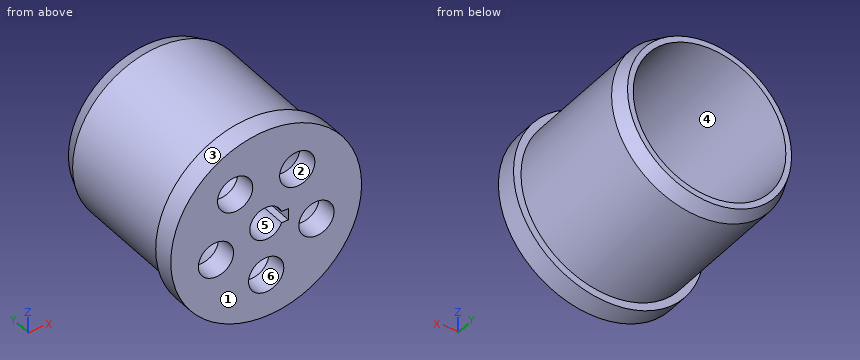
```python
from build123d import *

# Parameters (mm, degrees)
SKETCH1_R           = 41.275
SKETCH1_R_2         = 7.62
BOSS_EXTRUDE1_DEPTH = 9.525
SKETCH2_R           = 38.0365
SKETCH2_R_2         = 33.02
BOSS_EXTRUDE2_DEPTH = 63.5
SKETCH3_R           = 12.7
BOSS_EXTRUDE3_DEPTH = 15.875
CHAMFER1_SIZE       = 6.35
CHAMFER1_SIZE2      = 2.54
SKETCH4_R           = 12.7
BOSS_EXTRUDE4_DEPTH = 6.35
FILLET1_R           = 2.54


with BuildPart() as part:
    # Sketch1 → Boss-Extrude1 (new body)
    with BuildSketch(Plane(origin=(0, 0, 0), x_dir=(1, 0, 0), z_dir=(0, 1, 0))):
        Circle(SKETCH1_R)
        with Locations((-13.436770867, -18.494128491)):
            Circle(SKETCH1_R_2, mode=Mode.SUBTRACT)
        with Locations((13.436770867, -18.494128491)):
            Circle(SKETCH1_R_2, mode=Mode.SUBTRACT)
        with BuildLine():
            Line((9.6, -2.5), (6.64529909, -2.5))
            ThreePointArc((6.64529909, -2.5), (-7.1, 0), (6.64529909, 2.5))
            Line((6.64529909, 2.5), (9.6, 2.5))
            Line((9.6, 2.5), (9.6, -2.5))
        make_face(mode=Mode.SUBTRACT)
        with Locations((-21.741151963, 7.064128491)):
            Circle(SKETCH1_R_2, mode=Mode.SUBTRACT)
        with BuildLine():
            ThreePointArc((0, 15.24), (-7.62, 22.86), (0, 30.48))
            ThreePointArc((0, 30.48), (7.62, 22.86), (0, 15.24))
        make_face(mode=Mode.SUBTRACT)
        with Locations((21.741151963, 7.064128491)):
            Circle(SKETCH1_R_2, mode=Mode.SUBTRACT)
    extrude(amount=BOSS_EXTRUDE1_DEPTH)

    # Sketch2 → Boss-Extrude2 (add)
    with BuildSketch(Plane(origin=(0, 9.525, 0), x_dir=(1, 0, 0), z_dir=(0, 1, 0))):
        Circle(SKETCH2_R)
        Circle(SKETCH2_R_2, mode=Mode.SUBTRACT)
    extrude(amount=BOSS_EXTRUDE2_DEPTH)

    # Sketch3 → Boss-Extrude3 (add)
    with BuildSketch(Plane(origin=(0, 9.525, 0), x_dir=(1, 0, 0), z_dir=(0, 1, 0))):
        Circle(SKETCH3_R)
        with BuildLine():
            Line((9.6, -2.5), (6.64529909, -2.5))
            ThreePointArc((6.64529909, -2.5), (-7.1, 0), (6.64529909, 2.5))
            Line((6.64529909, 2.5), (9.6, 2.5))
            Line((9.6, 2.5), (9.6, -2.5))
        make_face(mode=Mode.SUBTRACT)
    extrude(amount=BOSS_EXTRUDE3_DEPTH)

    # Chamfer1
    chamfer1_edges = [part.edges().sort_by_distance(p)[0] for p in [
        (-38.0365, 73.025, 0),
    ]]
    chamfer1_side = [part.faces().sort_by_distance(p)[0] for p in [
        (-38.0365, 41.275, 0),
    ]]
    chamfer(chamfer1_edges, length=CHAMFER1_SIZE, length2=CHAMFER1_SIZE2, reference=chamfer1_side[0])

    # Sketch4 → Boss-Extrude4 (add)
    with BuildSketch(Plane(origin=(0, 25.4, 0), x_dir=(1, 0, 0), z_dir=(0, 1, 0))):
        Circle(SKETCH4_R)
    extrude(amount=BOSS_EXTRUDE4_DEPTH)

    # Fillet1
    fillet1_edges = [part.edges().sort_by_distance(p)[0] for p in [
        (-12.7, 31.75, 0),
    ]]
    fillet(fillet1_edges, radius=FILLET1_R)


solid = part.part
```
The listing builds one solid part. Answer for the finished solid, in the listing's coordinates (mm). Face numbers are marked on the shaded views. A direction names the side the tool comes from. Give positions to 0.01 mm unless a question says otherwise; leave off trailing zeros. Order: outer loops, then holes, each group sorted by start corner. A loop starts at its lowest first (then second) coordinate and runs counter-clockwise, first axis right, second up. Notation, with made-up numbers: (49, 26) - (85, 26) arc R25 ccw to (85, 41) - close; hole circle Ø7 at (37.5, -25). An arc over 180 degrees is marked (long way). Answer in a Markdown table with one row per item. Add a question column.
Q1. The part is cut by section D-D (z = 20.5). Give the number of separate pieces and of enclosed holes in the cut face, then the cut area to 3 significant figures.
Q2. The part is cut by section C-C (y = 28). Determine the outline of the cut face in (x, z), then the cut area to 3 significant figures.
Q3. For a pull along X with two mould halves and no side action, classify the marked faces 1, 2 and 3 as released by +X, released by -X, zero draft, split by the parting line, or undercut.
Q4. Find the intervals of material crossed by line 1 along Z through (x, y) = (0, 10.75); line 2 along Z through (x, y) = (19.5, 4); line 3 along X through (y, z) = (17, 2), in increasing order. Write a range as [from, to].
Q5. Given P1, Ø7, axis at x = 3, z = 0.5, coming from the -Y side; P2, Ø0.9, axis at x = 9, y = 9.5, coming from the -Z side; P3, Ø8, axis at x = -26, z = -5, coming from the +Y side (3 decimals); P4, Ø5.5, axis at y = 7, z = 1, coming from the -X side (3 decimals), each flat-ended and moving along its own axis, determine where each tip first touches the part or whether it passes through.
Q6. Which of the six approach directions +Z, -Z, +X, -X, +Y, -Y give full straight-line access (tool end or side, diameter ignored) to the marked faces 4, 5 and 6?
Q7. The part is cut by section A-A (y = 18). Determine the outline of the cut face in (x, z), then the cut area to 3 significant figures.
Determined:
| question | item | result |
|---|---|---|
| 1 | separate pieces | 3 |
| 1 | enclosed holes | 0 |
| 1 | area | 1,160 mm² |
| 2 | outline | circle Ø76.07 at (0, 0); circle Ø25.4 at (0, 0); hole circle Ø66.04 at (0, 0) |
| 2 | area | 1,630 mm² |
| 3 | face 1 | zero draft |
| 3 | face 2 | undercut |
| 3 | face 3 | split by the parting line |
| 4 | line 1 | z = [-38.04, -33.02], [-12.7, -7.1], [7.1, 12.7], [33.02, 38.04] |
| 4 | line 2 | z = [-36.38, -14.35], [0.22, 13.88], [23.11, 36.38] |
| 4 | line 3 | x = [-37.98, -32.96], [-12.54, -6.81], [9.6, 12.54], [32.96, 37.98] |
| 5 | P1 | stops at y = 25.4 |
| 5 | P2 | stops at z = -40.38 |
| 5 | P3 | stops at y = 9.525 |
| 5 | P4 | stops at x = -41.275 |
| 6 | face 4 | +Y |
| 6 | face 5 | -Y |
| 6 | face 6 | +Y, -Y |
| 7 | outline | circle Ø76.07 at (0, 0); circle Ø25.4 at (0, 0); hole circle Ø66.04 at (0, 0); hole (6.65, -2.5) - (9.6, -2.5) - (9.6, 2.5) - (6.65, 2.5) arc R7.1 ccw (long way) to start |
| 7 | area | 1,450 mm² |
